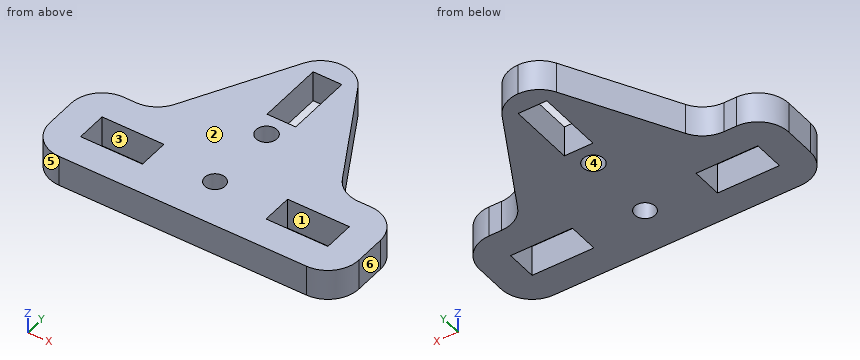
from build123d import *

# Parameters (mm, degrees)
SKETCH1_W           = 63.5
SKETCH1_H           = 19.05
BOSS_EXTRUDE1_DEPTH = 6.35
SKETCH2_R           = 2.0955
SKETCH2_W           = 12.7
SKETCH2_H           = 6.35
CUT_EXTRUDE1_DEPTH  = 6.35
BOSS_EXTRUDE2_DEPTH = 6.35
SKETCH4_R           = 2.159
SKETCH4_W           = 5.8928
SKETCH4_H           = 13.6271
CUT_EXTRUDE3_DEPTH  = 6.35
FILLET1_R           = 6.35


with BuildPart() as part:
    # Sketch1 → Boss-Extrude1 (new body)
    with BuildSketch(Plane.XY):
        Rectangle(SKETCH1_W, SKETCH1_H)
    extrude(amount=BOSS_EXTRUDE1_DEPTH)

    # Sketch2 → Cut-Extrude1 (cut)
    with BuildSketch(Plane.XY.offset(6.35)):
        Circle(SKETCH2_R)
        with Locations((-19.05, 0)):
            Rectangle(SKETCH2_W, SKETCH2_H)
        with Locations((19.05, 0)):
            Rectangle(SKETCH2_W, SKETCH2_H)
    extrude(amount=-CUT_EXTRUDE1_DEPTH, mode=Mode.SUBTRACT)

    # Sketch3 → Boss-Extrude2 (add)
    with BuildSketch(Plane.XY.offset(6.35)):
        with BuildLine():
            Line((-19.05, 9.525), (0, 9.525))
            Line((0, 9.525), (0, 24.839121342))
            ThreePointArc((0, 24.839121342), (-5.460357863, 27.947672283), (-5.574636807, 34.229832521))
            Line((-5.574636807, 34.229832521), (-19.05, 9.525))
        make_face()
        with BuildLine():
            ThreePointArc((-5.574636807, 34.229832521), (-5.460357863, 27.947672283), (0, 24.839121342))
            Line((0, 24.839121342), (0, 37.539121342))
            ThreePointArc((0, 37.539121342), (-3.24144906, 36.649479205), (-5.574636807, 34.229832521))
        make_face()
        with BuildLine():
            Line((0, 37.539121342), (0, 24.839121342))
            ThreePointArc((0, 24.839121342), (4.490128061, 26.698993282), (6.35, 31.189121342))
            ThreePointArc((6.35, 31.189121342), (6.15310672, 32.758126662), (5.574636947, 34.229832265))
            ThreePointArc((5.574636947, 34.229832265), (3.241449185, 36.649479131), (0, 37.539121342))
        make_face()
        with BuildLine():
            Line((0, 24.839121342), (0, 9.525))
            Line((0, 9.525), (19.05, 9.525))
            Line((19.05, 9.525), (5.574636947, 34.229832265))
            ThreePointArc((5.574636947, 34.229832265), (6.15310672, 32.758126662), (6.35, 31.189121342))
            ThreePointArc((6.35, 31.189121342), (4.490128061, 26.698993282), (0, 24.839121342))
        make_face()
    extrude(amount=-BOSS_EXTRUDE2_DEPTH)

    # Sketch4 → Cut-Extrude3 (cut)
    with BuildSketch(Plane(origin=(0, 0, 0), x_dir=(-1, 0, 0), z_dir=(0, 0, -1))):
        with Locations((0, 15.24)):
            Circle(SKETCH4_R)
        with Locations((0, 26.449976884)):
            Rectangle(SKETCH4_W, SKETCH4_H)
    extrude(amount=-CUT_EXTRUDE3_DEPTH, mode=Mode.SUBTRACT)

    # Fillet1
    fillet1_edges = [part.edges().sort_by_distance(p)[0] for p in [
        (31.75, -9.525, 3.175),
        (31.75, 9.525, 3.175),
        (19.05, 9.525, 3.175),
        (-31.75, -9.525, 3.175),
        (-31.75, 9.525, 3.175),
        (-19.05, 9.525, 3.175),
    ]]
    fillet(fillet1_edges, radius=FILLET1_R)


solid = part.part
Input: part model. Units: mm. Frame: model coordinates. Face numbers are marked on the shaded views. A direction names the side the tool comes from. Coordinates: 2 decimals unless noted, no trailing zeros. Order: outer loops, then holes, each group sorted by start corner. A loop starts at its lowest first (then second) coordinate and runs counter-clockwise, first axis right, second up. Notation, with made-up numbers: M 89,-12.5 L 93,-12.5 A15 ccw 93,4.5 Z; hole C 67.5,-1 d10. An arc over 180 degrees is marked long. Answer as CSV lines item,"result".
1. Section D-D (x = -4). Return the cut outline in (y, z) (3 decimals), then the cut area to 3 significant figures.
Reported:
outline,"M -9.525,0 L 36.121,0 L 36.121,6.35 L -9.525,6.35 Z"
area,"290 mm2"
2. Section C-C (y = 27.5). Return the cut outline in (x, z).
Reported:
outline,"M -9.25,0 L -2.95,0 L -2.95,6.35 L -9.25,6.35 Z; M 2.95,0 L 9.25,0 L 9.25,6.35 L 2.95,6.35 Z"
3. First-contact query: P1, Ø3, axis at x = -24.5, z = 2, coming from the +Y side (3 decimals); P2, Ø1.9, axis at y = 28.5, z = 3, coming from the +X side; P3, Ø1.9, axis at x = -18, z = 2.5, coming from the +Y side. Flat tips, straight axial feed; report the tip coordinate or a pass-through.
Reported:
P1,"y = 9.525"
P2,"x = 9.22"
P3,"y = 13.19"
4. Section B-B (z = 2.75). State how many separate pieces and enclosed holes the cut face has, then the cut area to 3 significant figures.
Reported:
separate pieces,"1"
enclosed holes,"5"
area,"1,540 mm2"
5. Material intervals for line 1 (X direction, y = 3, z = 0.75); line 2 (X direction, y = 27, z = 3); line 3 (X direction, y = 30, z = 4.75), sorted ascending. Write a range as from..to.
Reported:
line 1,"-31.75..-25.4, -12.7..12.7, 25.4..31.75"
line 2,"-9.52..-2.95, 2.95..9.52"
line 3,"-7.88..-2.95, 2.95..7.88"
6. Access query for the marked faces 1 and 2. Directions: +Z, -Z, +X, -X, +Y, -Y. A direction counts if a zero-diameter tool reaches every point of the face in a straight line with its end or side. Return the directions, or none.
Reported:
face 1,"+Z, -Z"
face 2,"+Z, +X, -X, +Y, -Y"
7. Section A-A (y = 0). Return the cut outline in (x, z), then the cut area to 3 significant figures.
Reported:
outline,"M -31.75,0 L -25.4,0 L -25.4,6.35 L -31.75,6.35 Z; M -12.7,0 L -2.1,0 L -2.1,6.35 L -12.7,6.35 Z; M 2.1,0 L 12.7,0 L 12.7,6.35 L 2.1,6.35 Z; M 25.4,0 L 31.75,0 L 31.75,6.35 L 25.4,6.35 Z"
area,"215 mm2"
8. Pull-direction query (Y, two-part tool) for the marked faces 3, 4, 5 and 6; classes: released by +Y, released by -Y, zero draft, split by the parting line, or undercut.
Reported:
face 3,"undercut"
face 4,"undercut"
face 5,"released by -Y"
face 6,"zero draft"
